Source: CAD feature listing. Evaluate the final solid. Frame: model axes, mm. A direction names the side the tool comes from. Give positions to 0.01 mm unless a question says otherwise; leave off trailing zeros. Order: outer loops, then holes, each group sorted by start corner. A loop starts at its lowest first (then second) coordinate and runs counter-clockwise, first axis right, second up. Notation, with made-up numbers: M 42,-34 L 63,-34 A28 ccw 63,-8 Z; hole C -9,15 d10. An arc over 180 degrees is marked long. Answer in a Markdown table with one row per item. Add a question column.
(1) Section query D-D, the plane y = 20. Return loops of the section in (x, z).
(2) Pin query (flat end, axial travel): P1, Ø5, axis at x = 58.5, z = -18, coming from the +Y side; P2, Ø15.5, axis at x = 87, z = -49.5, coming from the +Y side; P3, Ø0.9, axis at y = 37.5, z = -54.5, coming from the -X side; P4, Ø1.6, axis at x = 104.5, z = -35, coming from the +Y side. Return the tip coordinate at first contact, or that it passes through.
(3) Section query C-C, the plane z = -51. Return loops of the section in (x, y).
(4) Material intervals for line 1 along Z through (x, y) = (62, 0.5); line 2 along X through (y, z) = (6, -18.5); line 3 along X through (y, z) = (7.5, -42), sorted ascending.
(5) Set-up query: faces 1 (the face through (105.25, 38, 1)), 2 (the face through (91, 6, -39)), 3 (the face through (0, 38, -57)), 4 (the face through (106, 13, -27)). Return all of +Z, -Z, +X, -X, +Y, -Y with unobstructed straight access to the full face (end or side cutting, diameter ignored); none if empty.
(6) Section query B-B, the plane x = 10. Return loops of the section in (y, z), plus the area to 3 significant figures.
(7) Mould query, pull axis Y, two halves, no side actions, for faces 5 (the face through (52, 39.2, 1)), 6 (the face through (53, 41, 2)), 7 (the face through (52, 38, -56)), 8 (the face through (0, 38, 4)). Classes: pulls with the +Y half, pulls with the -Y half, needs draft (parallel to the pull), parting line crosses it, or undercut.
(8) Section query A-A, the plane y = 10. Return loops of the section in (x, z).
from build123d import *

# Parameters (mm, degrees)
SKETCH2_W           = 109
SKETCH2_H           = 65
SKETCH2_W_2         = 104
SKETCH2_H_2         = 53
SKETCH2_W_3         = 25
SKETCH2_H_3         = 14
BOSS_EXTRUDE1_DEPTH = 41
SKETCH3_W           = 109
SKETCH3_H           = 65
BOSS_EXTRUDE2_DEPTH = 5
SKETCH4_W           = 65
SKETCH4_H           = 6
CUT_EXTRUDE1_DEPTH  = 3
SKETCH5_W           = 25
SKETCH5_H           = 18
CUT_EXTRUDE2_DEPTH  = 10
SKETCH6_W           = 53
SKETCH6_H           = 28
CUT_EXTRUDE3_DEPTH  = 25
SKETCH7_W           = 3
SKETCH7_H           = 3.2
CUT_EXTRUDE4_DEPTH  = 105.25
SKETCH8_W           = 53
SKETCH8_H           = 4.2
CUT_EXTRUDE5_DEPTH  = 1


with BuildPart() as part:
    # Sketch2 → Boss-Extrude1 (new body)
    # profile 1 of 3: a face of its own
    with BuildSketch(Plane(origin=(0, 0, 0), x_dir=(1, 0, 0), z_dir=(0, 1, 0))):
        with Locations((51.5, 26.5)):
            Rectangle(SKETCH2_W, SKETCH2_H)
        with Locations((52, 26.5)):
            Rectangle(SKETCH2_W_2, SKETCH2_H_2, mode=Mode.SUBTRACT)
    # profile 2 of 3: a face of its own
    with BuildSketch(Plane(origin=(0, 0, 0), x_dir=(1, 0, 0), z_dir=(0, 1, 0))):
        with Locations((91.5, 46)):
            Rectangle(SKETCH2_W_3, SKETCH2_H_3)
    # profile 3 of 3: a face of its own
    with BuildSketch(Plane(origin=(0, 0, 0), x_dir=(1, 0, 0), z_dir=(0, 1, 0))):
        with Locations((91.5, 7)):
            Rectangle(SKETCH2_W_3, SKETCH2_H_3)
    extrude(amount=BOSS_EXTRUDE1_DEPTH)

    # Sketch3 → Boss-Extrude2 (add)
    with BuildSketch(Plane.XZ):
        with Locations((51.5, -26.5)):
            Rectangle(SKETCH3_W, SKETCH3_H)
    extrude(amount=BOSS_EXTRUDE2_DEPTH)

    # Sketch4 → Cut-Extrude1 (cut)
    with BuildSketch(Plane.ZY.offset(3)):
        with Locations((-26.5, 38)):
            Rectangle(SKETCH4_W, SKETCH4_H)
    extrude(amount=-CUT_EXTRUDE1_DEPTH, mode=Mode.SUBTRACT)

    # Sketch5 → Cut-Extrude2 (cut)
    with BuildSketch(Plane(origin=(106, 0, 0), x_dir=(0, 0, -1), z_dir=(1, 0, 0))):
        with Locations((30.75, 32)):
            Rectangle(SKETCH5_W, SKETCH5_H)
    extrude(amount=-CUT_EXTRUDE2_DEPTH, mode=Mode.SUBTRACT)

    # Sketch6 → Cut-Extrude3 (cut)
    with BuildSketch(Plane.ZY.offset(-79)):
        with Locations((-26.5, 27)):
            Rectangle(SKETCH6_W, SKETCH6_H)
    extrude(amount=-CUT_EXTRUDE3_DEPTH, mode=Mode.SUBTRACT)

    # Sketch7 → Cut-Extrude4 (cut)
    with BuildSketch(Plane.ZY):
        with Locations((-54.5, 37.6)):
            Rectangle(SKETCH7_W, SKETCH7_H)
        with Locations((1.5, 37.6)):
            Rectangle(SKETCH7_W, SKETCH7_H)
    extrude(amount=-CUT_EXTRUDE4_DEPTH, mode=Mode.SUBTRACT)

    # Sketch8 → Cut-Extrude5 (cut)
    with BuildSketch(Plane.ZY.offset(-104)):
        with Locations((-26.5, 38.1)):
            Rectangle(SKETCH8_W, SKETCH8_H)
    extrude(amount=-CUT_EXTRUDE5_DEPTH, mode=Mode.SUBTRACT)


solid = part.part
Values follow:
| question | item | result |
|---|---|---|
| 1 | outline | M -3,-59 L 106,-59 L 106,6 L -3,6 Z; hole M 0,-53 L 104,-53 L 104,0 L 0,0 Z |
| 2 | P1 | stops at y = 0 |
| 2 | P2 | stops at y = 41 |
| 2 | P3 | stops at x = 105.25 |
| 2 | P4 | stops at y = 23 |
| 3 | outline | M -3,-5 L 106,-5 L 106,41 L 104,41 L 104,40.2 L 105,40.2 L 105,36 L 104,36 L 104,13 L 79,13 L 79,0 L 0,0 L 0,35 L -3,35 Z |
| 4 | line 1 | z = -59 to -53, 0 to 6 |
| 4 | line 2 | x = -3 to 0, 104 to 106 |
| 4 | line 3 | x = -3 to 0, 79 to 106 |
| 5 | face 1 | -X |
| 5 | face 2 | +Y |
| 5 | face 3 | +Z, -Z, -X, +Y |
| 5 | face 4 | +Z, -Z, +X, +Y, -Y |
| 6 | outline | M -5,-59 L 41,-59 L 41,-53 L 39.2,-53 L 39.2,-56 L 36,-56 L 36,-53 L 0,-53 L 0,0 L 36,0 L 36,3 L 39.2,3 L 39.2,0 L 41,0 L 41,6 L -5,6 Z |
| 6 | area | 798 mm² |
| 7 | face 5 | undercut |
| 7 | face 6 | pulls with the +Y half |
| 7 | face 7 | undercut |
| 7 | face 8 | needs draft |
| 8 | outline | M -3,-59 L 106,-59 L 106,6 L -3,6 Z; hole M 0,-53 L 79,-53 L 79,-39 L 104,-39 L 104,-14 L 79,-14 L 79,0 L 0,0 Z |
